Geometry check sheet. Reference: the model listing, model coordinates, mm. Face numbers are marked on the shaded views. Coordinates: 2 decimals unless noted, no trailing zeros. Order: outer loops, then holes, each group sorted by start corner. A loop starts at its lowest first (then second) coordinate and runs counter-clockwise, first axis right, second up.
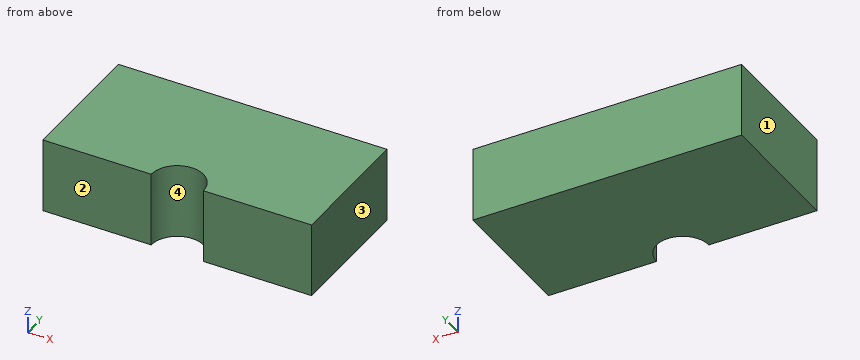
```python
from build123d import *

# Parameters (mm, degrees)
F1_DEPTH = 63.5


with BuildPart() as f1:
    # F0 (on Top) → F1 (new body)
    with BuildSketch(Plane.XY):
        with BuildLine():
            Line((114.3, 114.3), (-114.3, 114.3))
            Line((-114.3, 114.3), (-114.3, 0))
            Line((-114.3, 0), (-22.225, 0))
            ThreePointArc((-22.225, 0), (0, 22.225), (22.225, 0))
            Line((22.225, 0), (114.3, 0))
            Line((114.3, 0), (114.3, 114.3))
        make_face()
    extrude(amount=-F1_DEPTH)


solid = f1.part
```
Item 1: Sectioned sample at B-B (x = 0). Record the cut outline in (y, z) (3 decimals).
Item 2: Sectioned sample at A-A (z = -22). Record the cut outline in (x, y) (3 decimals), and give its area (3 significant figures).
Item 3: Depth check by flat-ended pin: P1, Ø6, axis at x = 9, y = 14.5, coming from the +Z side; P2, Ø10, axis at x = 17.5, y = 32.5, coming from the +Z side. Enter the tip coordinate at first touch or a pass-through.
Item 4: Thickness scan on line 1 along X through (y, z) = (11, -31); line 2 along X through (y, z) = (15.5, -57.5); line 3 along Y through (x, z) = (-4, -14). Record the ranges inside material, lowest first.
Item 5: Release check for a two-part mould opening along X. For the marked faces 1, 2, 3 and 4 record: pulls with the +X half, pulls with the -X half, needs draft (parallel to the pull), parting line crosses it, or undercut.
Geometry check:
1. outline: (22.225, -63.5) - (114.3, -63.5) - (114.3, 0) - (22.225, 0) - close
2. outline: (-114.3, 0) - (-22.225, 0) arc R22.225 cw to (22.225, 0) - (114.3, 0) - (114.3, 114.3) - (-114.3, 114.3) - close
2. area: 25,400 mm2
3. P1: passes through
3. P2: stops at z = 0
4. line 1: x = -114.3 to -19.31, 19.31 to 114.3
4. line 2: x = -114.3 to -15.93, 15.93 to 114.3
4. line 3: y = 21.86 to 114.3
5. face 1: pulls with the -X half
5. face 2: needs draft
5. face 3: pulls with the +X half
5. face 4: undercut
